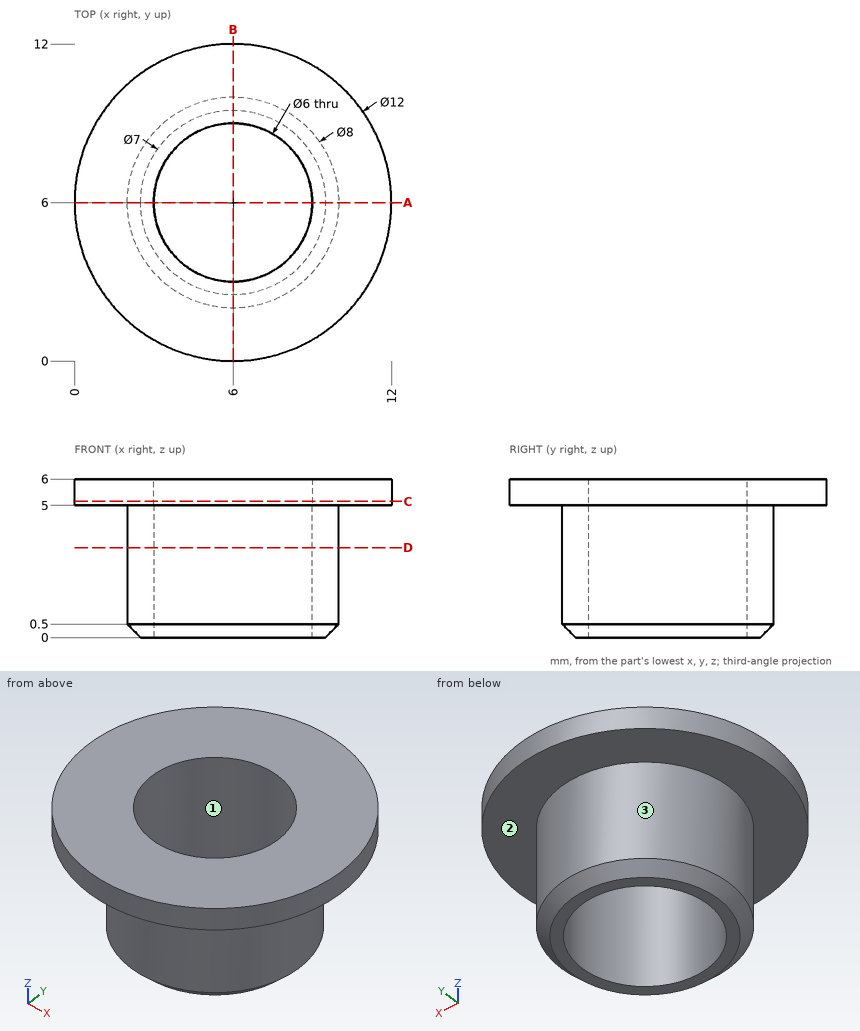
Geometry check sheet. Reference: drawing and pictorial views, mm from the part's lowest x, y, z. Coordinates: 2 decimals unless noted, no trailing zeros. Loops run counter-clockwise (first coordinate to the right, second up) from the corner with the lowest first, then second, coordinate; pieces in that order, holes last. Notation, with made-up numbers: (-1, -27) -> (25, -27) arc R21 cw to (25, -3) -> close; hole circle Ø11 at (73, -17.5). An arc over 180 degrees is marked (long way). Put each result on its own line as item: value.
1) Cross-section at A-A on y = 6. Record the boundary of the cut face in (x, z).
Result set:
outline: (0, 5) -> (2, 5) -> (2, 0.5) -> (2.5, 0) -> (3, 0) -> (3, 6) -> (0, 6) -> close; (9, 0) -> (9.5, 0) -> (10, 0.5) -> (10, 5) -> (12, 5) -> (12, 6) -> (9, 6) -> close
2) Gauge pin test, flat ends, axial feed: pin 1 Ø2 at (x, z) = (3, 3.5) entering from +Y; pin 2 Ø1.5 at (x, z) = (8.5, 4) entering from +Y; pin 3 Ø2 at (y, z) = (9.5, 5) entering from +X. Record the tip position at first contact, or that the pin passes through.
Result set:
pin 1: stops at y = 9.46
pin 2: stops at y = 9.6
pin 3: stops at x = 11.45
3) Release check for a two-part mould opening along Y. For the marked faces 1, 2 and 3 record: released by +Y, released by -Y, zero draft, split by the parting line, or undercut.
Result set:
face 1: undercut
face 2: zero draft
face 3: split by the parting line
4) Cross-section at C-C on z = 5.15. Record the boundary of the cut face in (x, y), plus the area to 3 significant figures.
Result set:
outline: circle Ø12 at (6, 6); hole circle Ø6 at (6, 6)
area: 84.8 mm^2
5) Cross-section at D-D on z = 3.4. Record the boundary of the cut face in (x, y), plus the area to 3 significant figures.
Result set:
outline: circle Ø8 at (6, 6); hole circle Ø6 at (6, 6)
area: 22.0 mm^2
6) Thickness scan on line 1 (Y direction, x = 6, z = 4.25); line 2 (Z direction, x = 9.75, y = 3.75); line 3 (X direction, y = 7, z = 2.6). Record the ranges inside material, lowest first.
Result set:
line 1: y = 2 to 3, 9 to 10
line 2: z = 5 to 6
line 3: x = 2.13 to 3.17, 8.83 to 9.87
